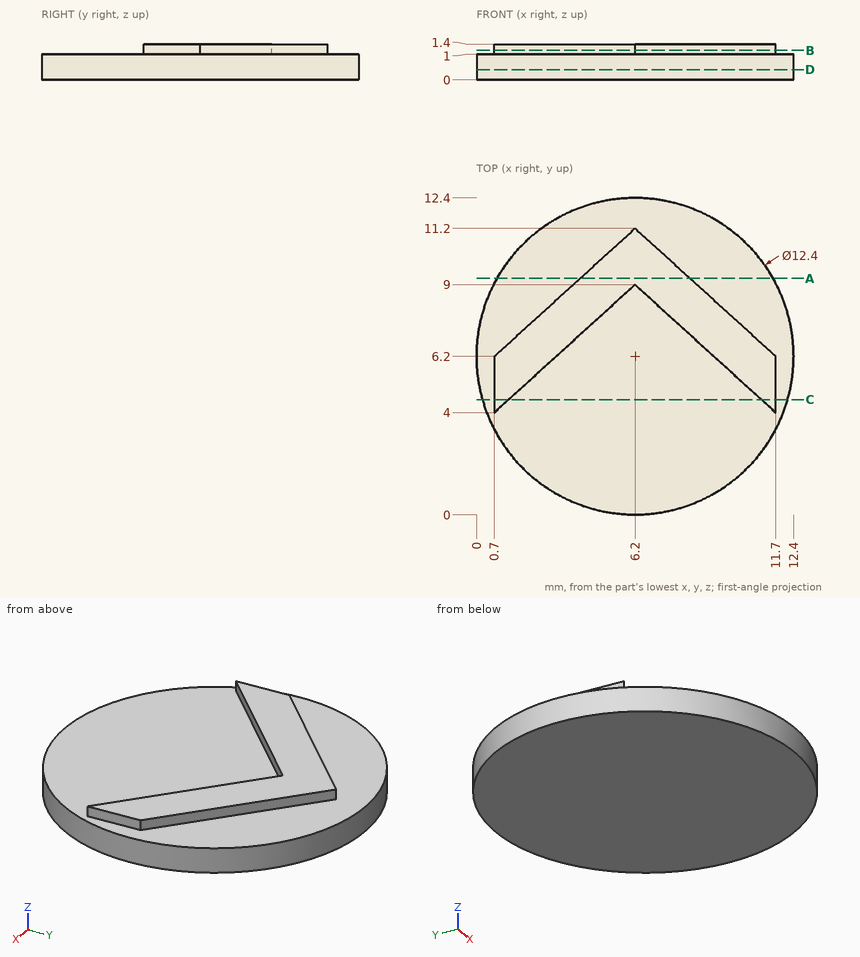
The figure shows three views and two pictorial views of one solid part (mm, origin at its lowest corner). Answer the questions. Round coordinates to 2 decimals unless told otherwise and drop trailing zeros. Order: outer loops, then holes, each group sorted by start corner. A loop starts at its lowest first (then second) coordinate and runs counter-clockwise, first axis right, second up. Notation, with made-up numbers: (8, -25.75) - (33, -25.75) arc R23 cw to (33, 6.25) - close; hole circle Ø9 at (87, 27). An arc over 180 degrees is marked (long way). Write item = value, one per line. Start each with the question number.
1) Straight lines are drawn through the part: L1, parallel to Z at x = 6.5, y = 11.25; L2, parallel to X at y = 8.75, z = 1.2 (3 decimals); L3, parallel to X at y = 6.5, z = 1.2. For each, find the intervals that lie inside material, in ascending order.
2) Section D-D, the plane z = 0.4 is taken. Write down the section's boundary in (x, y), plus the area to 3 significant figures.
3) Section C-C, the plane y = 4.5 is taken. Write down the section's boundary in (x, z).
4) Section A-A, the plane y = 9.25 is taken. Write down the section's boundary in (x, z) (3 decimals), plus the area to 3 significant figures.
5) Section B-B, the plane z = 1.15 is taken. Write down the section's boundary in (x, y).
Results list:
q1.L1 = 0 to 1
q1.L2 = 3.505 to 5.925, 6.475 to 8.895
q1.L3 = 1.03 to 3.45, 8.95 to 11.37
q2.outline = circle Ø12.4 at (6.2, 6.2)
q2.area = 121 mm^2
q3.outline = (0.24, 0) - (12.16, 0) - (12.16, 1) - (11.7, 1) - (11.7, 1.4) - (11.15, 1.4) - (11.15, 1) - (1.25, 1) - (1.25, 1.4) - (0.7, 1.4) - (0.7, 1) - (0.24, 1) - close
q4.outline = (0.802, 0) - (11.598, 0) - (11.598, 1) - (8.345, 1) - (8.345, 1.4) - (4.055, 1.4) - (4.055, 1) - (0.802, 1) - close
q4.area = 12.5 mm^2
q5.outline = (0.7, 4) - (6.2, 9) - (11.7, 4) - (11.7, 6.2) - (6.2, 11.2) - (0.7, 6.2) - close
